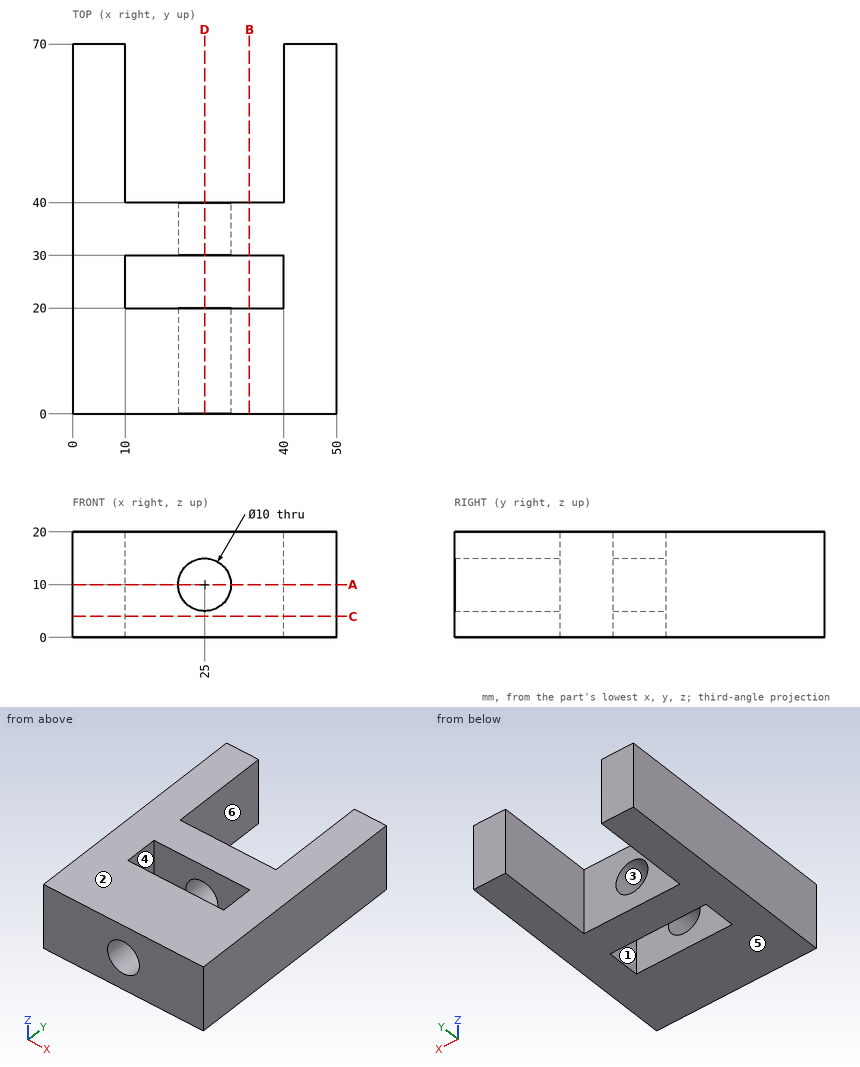
Geometry: see drawing. Coordinates: mm, zero at the bounding-box minimum. A direction names the side the tool comes from. Give positions to 0.01 mm unless a question says otherwise; leave off trailing zeros. Loops run counter-clockwise (first coordinate to the right, second up) from the corner with the lowest first, then second, coordinate; pieces in that order, holes last. Notation, with made-up numbers: (3.25, 84) -> (8.25, 84) arc R31 ccw to (8.25, 119) -> close; hole circle Ø7 at (57, -25.5). An arc over 180 degrees is marked (long way). Use one line per item in the form item = value.
Item 1: Pin query (flat end, axial travel): P1, Ø3, axis at x = 20.5, z = 8.5, coming from the +Y side. Return the tip coordinate at first contact, or that it passes through.
A:
P1 = 40
Item 2: Access query for the marked faces 4, 5 and 6. Directions: +Z, -Z, +X, -X, +Y, -Y. A direction counts if a zero-diameter tool reaches every point of the face in a straight line with its end or side. Return the directions, or none.
A:
face_4 = +Z, -Z
face_5 = -Z, +X, -X, +Y, -Y
face_6 = +Z, -Z, +Y
Item 3: Line query: probe 1 along Z at (x, y) = (25, 5); probe 2 along Y at (x, z) = (35, 13.75); probe 3 along X at (y, z) = (10.5, 9.75). Output: solid intervals per line, ascending.
A:
probe_1 = 0 to 5, 15 to 20
probe_2 = 0 to 20, 30 to 40
probe_3 = 0 to 20.01, 29.99 to 50
Item 4: Draft query along Z for the marked faces 1, 2 and 3. Return one class per face: pulls with the +Z half, pulls with the -Z half, needs draft (parallel to the pull), parting line crosses it, or undercut.
A:
face_1 = needs draft
face_2 = pulls with the +Z half
face_3 = undercut
Item 5: Section query D-D on x = 25. Output: boundary loops of the cut face in (y, z), and give its area (3 significant figures).
A:
outline = (0, 0) -> (20, 0) -> (20, 5) -> (0, 5) -> close; (0, 15) -> (20, 15) -> (20, 20) -> (0, 20) -> close; (30, 0) -> (40, 0) -> (40, 5) -> (30, 5) -> close; (30, 15) -> (40, 15) -> (40, 20) -> (30, 20) -> close
area = 300 mm^2
Item 6: Section query A-A on z = 10. Output: boundary loops of the cut face in (x, y), and give its area (3 significant figures).
A:
outline = (0, 0) -> (20, 0) -> (20, 20) -> (10, 20) -> (10, 30) -> (20, 30) -> (20, 40) -> (10, 40) -> (10, 70) -> (0, 70) -> close; (30, 0) -> (50, 0) -> (50, 70) -> (40, 70) -> (40, 40) -> (30, 40) -> (30, 30) -> (40, 30) -> (40, 20) -> (30, 20) -> close
area = 2,000 mm^2
Item 7: Section query C-C on z = 4. Output: boundary loops of the cut face in (x, y), and give its area (3 significant figures).
A:
outline = (0, 0) -> (50, 0) -> (50, 70) -> (40, 70) -> (40, 40) -> (10, 40) -> (10, 70) -> (0, 70) -> close; hole (10, 20) -> (40, 20) -> (40, 30) -> (10, 30) -> close
area = 2,300 mm^2
Item 8: Section query B-B on x = 33.5. Output: boundary loops of the cut face in (y, z), and give its area (3 significant figures).
A:
outline = (0, 0) -> (20, 0) -> (20, 20) -> (0, 20) -> close; (30, 0) -> (40, 0) -> (40, 20) -> (30, 20) -> close
area = 600 mm^2
